For this review, take the finished solid that the model builds, in its own axes (mm). Face numbers are marked on the shaded views. A direction names the side the tool comes from. Coordinates: 2 decimals unless noted, no trailing zeros. Order: outer loops, then holes, each group sorted by start corner. A loop starts at its lowest first (then second) coordinate and runs counter-clockwise, first axis right, second up. Notation, with made-up numbers: (61.25, 2.5) - (112.25, 2.5) arc R22 ccw to (112.25, 8.5) - close; hole circle Ø3 at (23.25, 3). An arc over 180 degrees is marked (long way). One line per item, written item: value. Start each with the question number.
(1) Clearance check with flat-ended pins moving along their axes: pin 1 (16.5 mm diameter, centred on x = 71.26, y = 55.74, fed in from +Z); pin 2 (20.5 mm diameter, centred on x = 132.5, z = 42.5, fed in from +Y); pin 3 (10.5 mm diameter, centred on x = 127.5, y = 14.5, fed in from +Z). State where each tip first meets the part, or that it passes through.
(2) For the marked faces 1, 2 and 3, list the 3-axis set-ups (+Z, -Z, +X, -X, +Y, -Y) from which the entire face can be reached by the end or side of a thin tool; tool diameter is ignored.
(3) Consider section A-A on x = 68.5. Write out the cut boundary in (y, z).
(4) To check wall thickness, follow line 1 along X through (y, z) = (55, 20); line 2 along Y through (x, z) = (130.5, 77); line 3 along X through (y, z) = (14, 82.5). State the ranges of each line that lie inside material, in increasing order.
(5) Consider section B-B on z = 69.85. Write out the cut boundary in (x, y), then the cut area to 3 significant figures.
(6) Consider section C-C on x = 34. Write out the cut boundary in (y, z).
(7) Consider section D-D on y = 52. Write out the cut boundary in (x, z), then the cut area to 3 significant figures.
```python
from build123d import *

# Parameters (mm, degrees)
F1_DEPTH  = 12.7
F3_DEPTH  = 25.4
F4_W      = 12.7
F4_H      = 120.65
F5_DEPTH  = 95.25
F7_DEPTH  = 25.4
F9_DEPTH  = 25.4
F11_DEPTH = 25.4
F12_W     = 41.275
F12_H     = 9.525
F13_DEPTH = 76.2
F15_DEPTH = 25.4
F17_DEPTH = 25.4
F19_DEPTH = 25.4
F21_DEPTH = 25.4
F23_DEPTH = 25.4
F24_R     = 19.05
F25_DEPTH = 25.4
F27_DEPTH = 25.4


with BuildPart() as f1:
    # F0 (on Top) → F1 (new body)
    with BuildSketch(Plane.XY):
        Polygon((20.463030386, 81.1401112616), (-62.086969614, -1.4098887384), (-62.086969614, -39.5098887384), (141.113030386, -39.5098887384), (160.163030386, -20.4598887384), (160.163030386, 81.1401112616), (71.263030386, 81.1401112616), (36.338030386, 81.1401112616), align=None)
    extrude(amount=F1_DEPTH)

    # F2 (on face) → F3 (cut)
    with BuildSketch(Plane.XY.offset(12.7)):
        Polygon((160.163030386, 62.0901112616), (160.163030386, 81.1401112616), (141.113030386, 81.1401112616), align=None)
    extrude(amount=-F3_DEPTH, mode=Mode.SUBTRACT)

    # F4 (on face) → F5 (join)
    with BuildSketch(Plane.XY.offset(12.7)):
        with Locations((112.538030386, 20.8151112616)):
            Rectangle(F4_W, F4_H)
        with Locations((29.988030386, 20.8151112616)):
            Rectangle(F4_W, F4_H)
    extrude(amount=F5_DEPTH)

    # F6 (on face) → F7 (cut)
    with BuildSketch(Plane(origin=(23.638030386, 0, 0), x_dir=(0, -1, 0), z_dir=(-1, 0, 0))):
        Polygon((-62.0901112616, 107.95), (-81.1401112616, 107.95), (-81.1401112616, 88.9), align=None)
    extrude(amount=-F7_DEPTH, mode=Mode.SUBTRACT)

    # F8 (on face) → F9 (cut)
    with BuildSketch(Plane(origin=(23.638030386, 0, 0), x_dir=(0, -1, 0), z_dir=(-1, 0, 0))):
        Polygon((39.5098887384, 107.95), (-23.9901112616, 107.95), (39.5098887384, 38.1), align=None)
    extrude(amount=-F9_DEPTH, mode=Mode.SUBTRACT)

    # F10 (on face) → F11 (cut)
    with BuildSketch(Plane.YZ.offset(118.888030386)):
        Polygon((-39.5098887384, 38.1), (23.9901112616, 107.95), (-39.5098887384, 107.95), align=None)
        Polygon((62.0901112616, 107.95), (81.1401112616, 88.9), (81.1401112616, 107.95), align=None)
    extrude(amount=-F11_DEPTH, mode=Mode.SUBTRACT)

    # F12 (on face) → F13 (join)
    with BuildSketch(Plane.XY.offset(12.7)):
        with Locations((139.525530386, 12.8776112616)):
            Rectangle(F12_W, F12_H)
    extrude(amount=F13_DEPTH)

    # F14 (on face) → F15 (cut)
    with BuildSketch(Plane.XZ.offset(-8.1151112616)):
        Polygon((160.163030386, 88.9), (131.588030386, 88.9), (160.163030386, 25.4), align=None)
    extrude(amount=-F15_DEPTH, mode=Mode.SUBTRACT)

    # F16 (on face) → F17 (cut)
    with BuildSketch(Plane.XY.offset(12.7)):
        with BuildLine():
            ThreePointArc((-49.386969614, -26.8098887384), (-43.036969614, -33.1598887384), (-36.686969614, -26.8098887384))
            ThreePointArc((-36.686969614, -26.8098887384), (-43.036969614, -20.4598887384), (-49.386969614, -26.8098887384))
        make_face()
    extrude(amount=-F17_DEPTH, mode=Mode.SUBTRACT)

    # F18 (on face) → F19 (cut)
    with BuildSketch(Plane.XY.offset(12.7)):
        with BuildLine():
            ThreePointArc((141.113030386, -26.8098887384), (145.6031584465, -24.9500167989), (147.463030386, -20.4598887384))
            ThreePointArc((147.463030386, -20.4598887384), (136.6229023254, -15.9697606779), (141.113030386, -26.8098887384))
        make_face()
    extrude(amount=-F19_DEPTH, mode=Mode.SUBTRACT)

    # F20 (on face) → F21 (cut)
    with BuildSketch(Plane.XY.offset(12.7)):
        with BuildLine():
            ThreePointArc((147.463030386, 55.7401112616), (145.6031584465, 60.2302393221), (141.113030386, 62.0901112616))
            ThreePointArc((141.113030386, 62.0901112616), (136.6229023254, 51.2499832011), (147.463030386, 55.7401112616))
        make_face()
    extrude(amount=-F21_DEPTH, mode=Mode.SUBTRACT)

    # F22 (on face) → F23 (cut)
    with BuildSketch(Plane.XY.offset(12.7)):
        with BuildLine():
            ThreePointArc((71.263030386, -14.1098887384), (64.913030386, -20.4598887384), (71.263030386, -26.8098887384))
            Line((71.263030386, -26.8098887384), (71.263030386, -20.4598887384))
            Line((71.263030386, -20.4598887384), (71.263030386, -14.1098887384))
        make_face()
        with BuildLine():
            ThreePointArc((77.613030386, 55.7401112616), (66.7729023254, 60.2302393221), (71.263030386, 49.3901112616))
            ThreePointArc((71.263030386, 49.3901112616), (75.7531584465, 51.2499832011), (77.613030386, 55.7401112616))
        make_face()
        with BuildLine():
            Line((71.263030386, -20.4598887384), (71.263030386, -26.8098887384))
            ThreePointArc((71.263030386, -26.8098887384), (75.7531584465, -24.9500167989), (77.613030386, -20.4598887384))
            ThreePointArc((77.613030386, -20.4598887384), (75.7531584465, -15.9697606779), (71.263030386, -14.1098887384))
            Line((71.263030386, -14.1098887384), (71.263030386, -20.4598887384))
        make_face()
    extrude(amount=-F23_DEPTH, mode=Mode.SUBTRACT)

    # F24 (on face) → F25 (cut)
    with BuildSketch(Plane.YZ.offset(118.888030386)):
        with Locations((43.0320575833, 69.85)):
            Circle(F24_R)
    extrude(amount=-F25_DEPTH, mode=Mode.SUBTRACT)

    # F26 (on face) → F27 (cut)
    with BuildSketch(Plane(origin=(23.638030386, 0, 0), x_dir=(0, -1, 0), z_dir=(-1, 0, 0))):
        with BuildLine():
            ThreePointArc((-62.0901112616, 69.85), (-43.0401112616, 50.8), (-23.9901112616, 69.85))
            ThreePointArc((-23.9901112616, 69.85), (-43.0401112616, 88.9), (-62.0901112616, 69.85))
        make_face()
    extrude(amount=-F27_DEPTH, mode=Mode.SUBTRACT)


solid = f1.part
```
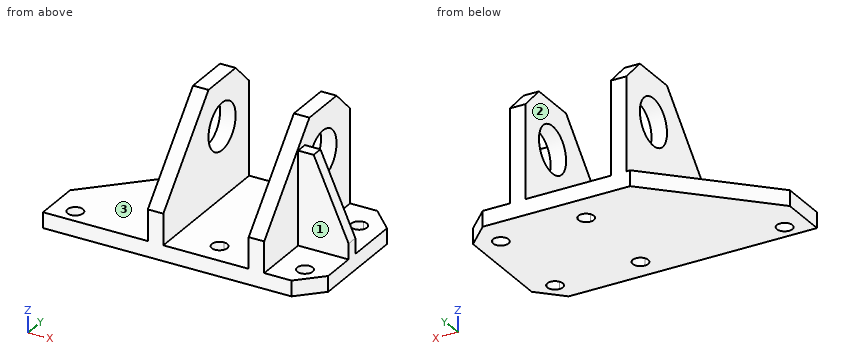
Geometry check:
1. pin 1: stops at z = 12.7
1. pin 2: stops at y = 17.64
1. pin 3: stops at z = 88.9
2. face 1: +Z, +X, -Y
2. face 2: +Z, +Y, -Y
2. face 3: +Z, -X, +Y, -Y
3. outline: (-39.51, 0) - (-26.18, 0) - (-26.18, 12.7) - (-39.51, 12.7) - close; (-14.74, 0) - (50.02, 0) - (50.02, 12.7) - (-14.74, 12.7) - close; (61.46, 0) - (81.14, 0) - (81.14, 12.7) - (61.46, 12.7) - close
4. line 1: x = 23.64 to 36.34, 106.19 to 118.89
4. line 2: y = 8.12 to 17.64
4. line 3: x = 23.64 to 36.34, 106.19 to 134.47
5. outline: (23.64, -10.65) - (36.34, -10.65) - (36.34, 23.99) - (23.64, 23.99) - close; (23.64, 62.09) - (36.34, 62.09) - (36.34, 81.14) - (23.64, 81.14) - close; (106.19, -10.65) - (118.89, -10.65) - (118.89, 8.12) - (140.16, 8.12) - (140.16, 17.64) - (118.89, 17.64) - (118.89, 23.98) - (106.19, 23.98) - close; (106.19, 62.08) - (118.89, 62.08) - (118.89, 81.14) - (106.19, 81.14) - close
5. area: 1,570 mm^2
6. outline: (-39.51, 0) - (81.14, 0) - (81.14, 88.9) - (62.09, 107.95) - (23.99, 107.95) - (-39.51, 38.1) - close; hole circle Ø38.1 at (43.04, 69.85)
7. outline: (-8.68, 0) - (66.13, 0) - (66.13, 12.7) - (36.34, 12.7) - (36.34, 53.04) - (23.64, 53.04) - (23.64, 12.7) - (-8.68, 12.7) - close; (23.64, 86.66) - (36.34, 86.66) - (36.34, 107.95) - (23.64, 107.95) - close; (76.39, 0) - (135.98, 0) - (135.98, 12.7) - (118.89, 12.7) - (118.89, 53.04) - (106.19, 53.04) - (106.19, 12.7) - (76.39, 12.7) - close; (106.19, 86.66) - (118.89, 86.66) - (118.89, 107.95) - (106.19, 107.95) - close; (146.24, 0) - (160.16, 0) - (160.16, 12.7) - (146.24, 12.7) - close
7. area: 3,450 mm^2
